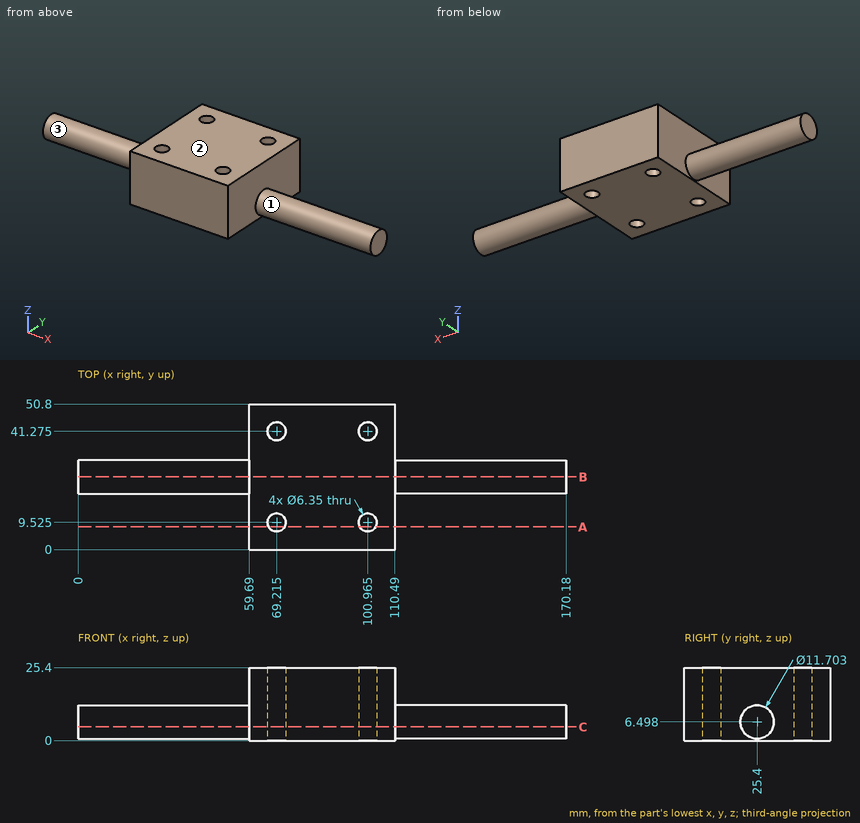
Answer from the drawing. Dimensions are ordinates in mm from the lowest x, y and z of the part. A direction names the side the tool comes from. Round coordinates to 2 decimals unless told otherwise and drop trailing zeros. Write each loop counter-clockwise with the first axis right and the second up, starting at its lowest first coordinate (ties: lowest second). Pieces come first, ordered by that corner, then holes. Notation, with made-up numbers: (35, 7) -> (88, 7) arc R36 ccw to (88, 41) -> close; hole circle Ø9 at (-24.5, -18). An arc over 180 degrees is marked (long way). Write each question's results on one line, items separated by ' | '.
1) Flat-ended cylindrical pins translate along their axes: pin 1 (6 mm diameter, centred on x = 17.5, z = 10, fed in from +Y); pin 2 (1.5 mm diameter, centred on x = 46, y = 31.5, fed in from -Z) (1 decimal); pin 3 (2 mm diameter, centred on x = 139, y = 26, fed in from +Z). Find the tip coordinate at first contact, or state that the pin passes through.
Findings:
pin 1: stops at y = 31.23 | pin 2: stops at z = 4.1 | pin 3: stops at z = 12.35
2) Consider line 1 along X through (y, z) = (15, 17.75); line 2 along Z through (x, y) = (33, 25) (1 decimal); line 3 along Y through (x, z) = (13.5, 9). Determine where each line is inside the solid, lowest interval first. Write a range as [from, to].
Findings:
line 1: x = [59.69, 110.49] | line 2: z = [0.7, 12.3] | line 3: y = [20.11, 30.69]
3) The part is cut by section A-A (y = 8). Write down the section's boundary in (x, z).
Findings:
outline: (59.69, 0) -> (66.43, 0) -> (66.43, 25.4) -> (59.69, 25.4) -> close; (72, 0) -> (98.18, 0) -> (98.18, 25.4) -> (72, 25.4) -> close; (103.75, 0) -> (110.49, 0) -> (110.49, 25.4) -> (103.75, 25.4) -> close
4) The part is cut by section C-C (z = 4.75). State how many separate pieces and enclosed holes the cut face has, and give its area (3 significant figures).
Findings:
separate pieces: 1 | enclosed holes: 4 | area: 3,790 mm²
5) The part is cut by section B-B (y = 25.4). Write down the section's boundary in (x, z), and give its area (3 significant figures).
Findings:
outline: (0, 0.65) -> (59.69, 0.65) -> (59.69, 0) -> (110.49, 0) -> (110.49, 0.65) -> (170.18, 0.65) -> (170.18, 12.35) -> (110.49, 12.35) -> (110.49, 25.4) -> (59.69, 25.4) -> (59.69, 12.35) -> (0, 12.35) -> close | area: 2,690 mm²
6) Which of the six approach directions +Z, -Z, +X, -X, +Y, -Y give full straight-line access (tool end or side, diameter ignored) to the marked faces 1, 2 and 3?
Findings:
face 1: +X | face 2: +Z, +X, -X, +Y, -Y | face 3: -X
